```python
from build123d import *

# Parameters (mm, degrees)
F1_DEPTH = 25.0000008
F2_R     = 2.54
F4_D     = 18
F6_D     = 4


with BuildPart() as f1:
    # F0 (on Right) → F1 (new body)
    with BuildSketch(Plane.YZ):
        Polygon((1, 86.2317622141), (0, 86.2317622141), (0, 57.2317622141), (-20, 57.2317622141), (-20, -2.7682377859), (0, -2.7682377859), (0, -31.7682377859), (1, -31.7682377859), (1, -1.7682377859), (-19, -1.7682377859), (-19, 56.2317622141), (1, 56.2317622141), align=None)
    extrude(amount=-F1_DEPTH)

    # F2
    f2_edges = [f1.edges().sort_by_distance(p)[0] for p in [
        (0, 0.5, 86.231762),
        (-25.000001, 0.5, 86.231762),
        (0, 0.5, -31.768238),
        (-25.000001, 0.5, -31.768238),
    ]]
    fillet(f2_edges, radius=F2_R)

    # F4 (through all)
    with Locations(Plane(origin=(0, 0, 0), x_dir=(1, 0, 0), z_dir=(0, 1, 0))):
        with Locations((-12.5000008, -27.2317622141)):
            Hole(F4_D / 2)

    # F6 (through all)
    with Locations(Plane.XZ):
        with Locations((-12.5000008, 73.7317622141), (-12.5, -19.2682377859)):
            Hole(F6_D / 2)


solid = f1.part
```
Model file for the job. Use its own axes, mm. A direction names the side the tool comes from. Coordinates: 2 decimals unless noted, no trailing zeros. Loops run counter-clockwise (first coordinate to the right, second up) from the corner with the lowest first, then second, coordinate; pieces in that order, holes last. Notation, with made-up numbers: (-39, -31.5) - (-5, -31.5) arc R26 ccw to (-5, -16.5) - close; hole circle Ø8 at (-15, 53.5). An arc over 180 degrees is marked (long way). Answer as a JSON object with one key per item and string values. Group by question number.
(1) Cut at A-A (y = -16). Give the cut face in (x, z), then the cut area to 3 significant figures.
(2) Cut at C-C (z = 19.5). Give the cut face in (x, y), then the cut area to 3 significant figures.
(3) Two-plate mould, pull along Z, no slides. Class faces 1 (the face through (-13.6, 0.5, 75.4)), 2 (the face through (-24.236, 0.493, 85.507)), 3 (the face through (-15, 0, 72)): released by +Z, released by -Z, zero draft, split by the parting line, or undercut.
(4) Flat gauge pins, fed straight in: pin 1 (3.5 mm diameter, centred on x = -12.5, z = -19.27, fed in from -Y); pin 2 (8 mm diameter, centred on x = -15, z = -11.5, fed in from -Y); pin 3 (5 mm diameter, centred on x = -7, z = 44, fed in from +Y); pin 4 (10 mm diameter, centred on x = -17.5, y = -13, fed in from +Z). Where does each tip first touch, or does it go through?
(5) Cut at D-D (z = -6). Give the cut face in (x, y), then the cut area to 3 significant figures.
(6) Tool access for faces 4 (the face through (-12, 1, -17)), 5 (the face through (-12, -10, 57.232)), 6 (the face through (-12, -9, 56.232)), 7 (the face through (-12, 0, -17)): list every direction of +Z, -Z, +X, -X, +Y, -Y with a clear straight run to the whole face (end or side of a thin tool).
(7) Cut at B-B (x = -11.5). Give the cut face in (y, z).
(8) Probe line 1 along Z through (x, y) = (-12.5, -19.7); line 2 along Z through (x, y) = (-6.5, -13); line 3 along Z through (x, y) = (-12.5, 0.55). List the from-to ranges inside material, lowest first.
Geometry says:
{
 "1": {"outline": "(-25, -2.77) - (0, -2.77) - (0, -1.77) - (-25, -1.77) - close; (-25, 56.23) - (0, 56.23) - (0, 57.23) - (-25, 57.23) - close", "area": "50.0 mm^2"},
 "2": {"outline": "(-25, -20) - (-17.11, -20) - (-17.11, -19) - (-25, -19) - close; (-7.89, -20) - (0, -20) - (0, -19) - (-7.89, -19) - close", "area": "15.8 mm^2"},
 "3": {"face 1": "undercut", "face 2": "released by +Z", "face 3": "zero draft"},
 "4": {"pin 1": "passes through", "pin 2": "stops at y = 0", "pin 3": "stops at y = -19", "pin 4": "stops at z = 57.23"},
 "5": {"outline": "(-25, 0) - (0, 0) - (0, 1) - (-25, 1) - close", "area": "25.0 mm^2"},
 "6": {"face 4": "+Z, -Z, +X, -X, +Y", "face 5": "+Z, +X, -X, -Y", "face 6": "+X, -X, +Y", "face 7": "-Z, +X, -X, -Y"},
 "7": {"outline": "(-20, -2.77) - (0, -2.77) - (0, -17.54) - (1, -17.54) - (1, -1.77) - (-19, -1.77) - (-19, 18.29) - (-20, 18.29) - close; (-20, 36.18) - (-19, 36.18) - (-19, 56.23) - (1, 56.23) - (1, 72) - (0, 72) - (0, 57.23) - (-20, 57.23) - close; (0, -31.77) - (1, -31.77) - (1, -21) - (0, -21) - close; (0, 75.46) - (1, 75.46) - (1, 86.23) - (0, 86.23) - close"},
 "8": {"line 1": "z = -2.77 to 18.23, 36.23 to 57.23", "line 2": "z = -2.77 to -1.77, 56.23 to 57.23", "line 3": "z = -31.77 to -21.27, -17.27 to -1.77, 56.23 to 71.73, 75.73 to 86.23"}
}
